Check sheet for the modelled part. Datum: model origin and axes. Units: mm. Give positions to 0.01 mm unless a question says otherwise; leave off trailing zeros. Write each loop counter-clockwise with the first axis right and the second up, starting at its lowest first coordinate (ties: lowest second). Pieces come first, ordered by that corner, then holes. Notation, with made-up numbers: M -26,51.5 L -1,51.5 A23 cw -1,65.5 Z; hole C 86,64 d1. An arc over 180 degrees is marked long. One line per item, written item: value. Start each with the question number.
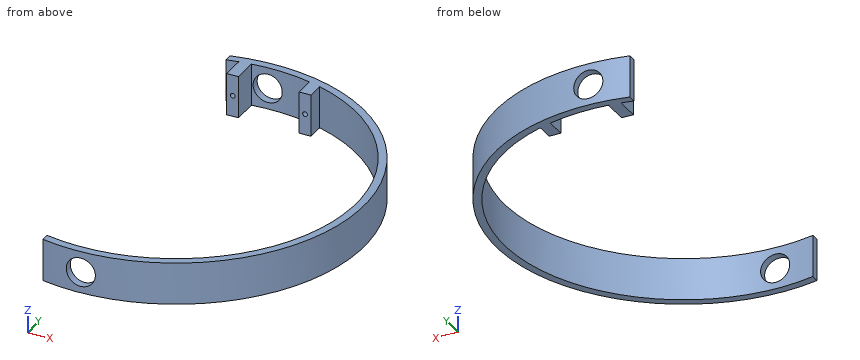
from build123d import *

# Parameters (mm, degrees)
BOSS_EXTRUDE1_DEPTH = 16
SKETCH2_R           = 5.5
CUT_EXTRUDE1_DEPTH  = 143
SKETCH3_W           = 4.5
SKETCH3_H           = 9.432893418
SKETCH3_H_2         = 7.692032902
BOSS_EXTRUDE2_DEPTH = 16
SKETCH4_R           = 0.9
CUT_EXTRUDE2_DEPTH  = 8


with BuildPart() as part:
    # Sketch1 → Boss-Extrude1 (new body)
    with BuildSketch(Plane.XY):
        with BuildLine():
            Line((-15, 140.397406292), (-15, 137.324957595))
            ThreePointArc((-15, 137.324957595), (68, 71), (-15, 4.675042405))
            Line((-15, 4.675042405), (-15, 1.602593708))
            ThreePointArc((-15, 1.602593708), (71, 71), (-15, 140.397406292))
        make_face()
    extrude(amount=BOSS_EXTRUDE1_DEPTH)

    # Sketch2 → Cut-Extrude1 (cut, through all)
    with BuildSketch(Plane(origin=(0, 0, 0), x_dir=(1, 0, 0), z_dir=(0, 1, 0))):
        with Locations((0, -8)):
            Circle(SKETCH2_R)
    extrude(amount=CUT_EXTRUDE1_DEPTH, mode=Mode.SUBTRACT)

    # Sketch3 → Boss-Extrude2 (add)
    with BuildSketch(Plane.XY.offset(16)):
        with Locations((-8.35, 133.916446709)):
            Rectangle(SKETCH3_W, SKETCH3_H)
        with Locations((19.05, 133.046016451)):
            Rectangle(SKETCH3_W, SKETCH3_H_2)
    extrude(amount=-BOSS_EXTRUDE2_DEPTH)

    # Sketch4 → Cut-Extrude2 (cut)
    with BuildSketch(Plane.XZ.offset(-129.2)):
        with Locations((19, 8)):
            Circle(SKETCH4_R)
        with Locations((-8.3, 8)):
            Circle(SKETCH4_R)
    extrude(amount=-CUT_EXTRUDE2_DEPTH, mode=Mode.SUBTRACT)


solid = part.part
1) Cross-section at C-C (x = 43). Record the boundary of the cut face in (y, z), plus the area to 3 significant figures.
2) Cross-section at D-D (y = 115). Record the boundary of the cut face in (x, z).
3) Cross-section at A-A (x = 0). Record the boundary of the cut face in (y, z).
4) Gauge pin test, flat ends, axial feed: pin 1 (4 mm diameter, centred on y = 63, z = 6, fed in from +X); pin 2 (1 mm diameter, centred on y = 74.5, z = 2.5, fed in from +X); pin 3 (5 mm diameter, centred on x = 19, z = 6, fed in from -Y). Record the tip position at first contact, or that the pin passes through.
5) Cross-section at B-B (z = 10.25). Record the boundary of the cut face in (x, y), plus the area to 3 significant figures.
6) Material ranges on L1, parallel to Z at x = 0, y = 2; L2, parallel to Z at x = 19, y = 133; L3, parallel to Y at x = 22, z = 4.5, recorded low to high. Write a range as from..to.
Data:
1. outline: M 14.5,0 L 18.32,0 L 18.32,16 L 14.5,16 Z; M 123.68,0 L 127.5,0 L 127.5,16 L 123.68,16 Z
1. area: 122 mm2
2. outline: M 51.85,0 L 55.72,0 L 55.72,16 L 51.85,16 Z
3. outline: M 0,0 L 3,0 L 3,2.5 L 0,2.5 Z; M 0,13.5 L 3,13.5 L 3,16 L 0,16 Z; M 139,0 L 142,0 L 142,2.5 L 139,2.5 Z; M 139,13.5 L 142,13.5 L 142,16 L 139,16 Z
4. pin 1: stops at x = 70.75
4. pin 2: stops at x = 70.94
4. pin 3: stops at y = 1.94
5. outline: M -15,1.6 A71 ccw -5.02,0.18 L -5.02,3.19 A68 cw -15,4.68 Z; M -15,137.32 A68 cw -10.6,138.17 L -10.6,129.2 L -6.1,129.2 L -6.1,138.63 L -7.06,138.63 A68 cw -5.02,138.81 L -5.02,141.82 A71 ccw -15,140.4 Z; M 5.02,0.18 A71 ccw 5.02,141.82 L 5.02,138.81 A68 cw 16.8,136.89 L 16.8,129.2 L 21.3,129.2 L 21.3,135.58 A68 cw 5.02,3.19 Z
5. area: 759 mm2
6. L1: z = 0..2.5, 13.5..16
6. L2: z = 0..7.1, 8.9..16
6. L3: y = 3.49..6.66, 135.34..138.51
